```python
from build123d import *

# Parameters (mm, degrees)
F1_DEPTH  = 38.1
F2_W      = 25.4
F2_H      = 38.1
F3_DEPTH  = 25.4
F4_R      = 6.35
F5_DEPTH  = 12.7
F7_DEPTH  = 12.7
F8_W      = 12.7
F8_H      = 12.7
F9_DEPTH  = 12.7
F11_DEPTH = 12.7
F12_R     = 1.5875
F13_DEPTH = 6.35
F15_DEPTH = 6.35


with BuildPart() as f1:
    # F0 (on Front) → F1 (new body)
    with BuildSketch(Plane.XZ):
        Polygon((-17.457331, 44.45), (-42.857331, 44.45), (-42.857331, 0), (26.992669, 0), (26.992669, 6.35), (-17.457331, 6.35), align=None)
    extrude(amount=F1_DEPTH)

    # F2 (on face) → F3 (cut)
    with BuildSketch(Plane.XZ.offset(38.1)):
        with Locations((-30.157331, 25.4)):
            Rectangle(F2_W, F2_H)
    extrude(amount=-F3_DEPTH, mode=Mode.SUBTRACT)

    # F4 (on face) → F5 (cut)
    with BuildSketch(Plane.XZ.offset(12.7)):
        with Locations((-30.157331, 31.75)):
            Circle(F4_R)
    extrude(amount=-F5_DEPTH, mode=Mode.SUBTRACT)

    # F6 (on face) → F7 (cut)
    with BuildSketch(Plane.XZ.offset(12.7)):
        with BuildLine():
            ThreePointArc((-42.857331, 31.75), (-39.137587, 40.730256), (-30.157331, 44.45))
            Line((-30.157331, 44.45), (-42.857331, 44.45))
            Line((-42.857331, 44.45), (-42.857331, 31.75))
        make_face()
        with BuildLine():
            Line((-17.457331, 44.45), (-30.157331, 44.45))
            ThreePointArc((-30.157331, 44.45), (-21.177075, 40.730256), (-17.457331, 31.75))
            Line((-17.457331, 31.75), (-17.457331, 44.45))
        make_face()
    extrude(amount=-F7_DEPTH, mode=Mode.SUBTRACT)

    # F8 (on face) → F9 (join)
    with BuildSketch(Plane.XZ.offset(12.7)):
        with Locations((-11.107331, 12.7)):
            Rectangle(F8_W, F8_H)
    extrude(amount=-F9_DEPTH)

    # F10 (on face) → F11 (cut)
    with BuildSketch(Plane.XZ.offset(12.7)):
        with BuildLine():
            Line((-4.757331, 19.05), (-17.457331, 19.05))
            ThreePointArc((-17.457331, 19.05), (-13.737587, 10.069744), (-4.757331, 6.35))
            Line((-4.757331, 6.35), (-4.757331, 19.05))
        make_face()
    extrude(amount=-F11_DEPTH, mode=Mode.SUBTRACT)

    # F12 (on face) → F13 (cut)
    with BuildSketch(Plane.XY.offset(6.35)):
        with Locations((-33.332331, -28.575)):
            Circle(F12_R)
        with Locations((17.467669, -28.575)):
            Circle(F12_R)
        with Locations((17.467669, -9.525)):
            Circle(F12_R)
    extrude(amount=-F13_DEPTH, mode=Mode.SUBTRACT)

    # F14 (on face) → F15 (cut)
    with BuildSketch(Plane.XY.offset(6.35)):
        with BuildLine():
            ThreePointArc((-30.157331, -38.1), (-39.137587, -34.380256), (-42.857331, -25.4))
            Line((-42.857331, -25.4), (-42.857331, -38.1))
            Line((-42.857331, -38.1), (-30.157331, -38.1))
        make_face()
        with BuildLine():
            ThreePointArc((26.992669, -25.4), (23.272925, -34.380256), (14.292669, -38.1))
            Line((14.292669, -38.1), (26.992669, -38.1))
            Line((26.992669, -38.1), (26.992669, -25.4))
        make_face()
    extrude(amount=-F15_DEPTH, mode=Mode.SUBTRACT)


solid = f1.part
```
Read the model definition and answer for the solid it produces. Units are mm, in the model's axes. A direction names the side the tool comes from. Coordinates: 2 decimals unless noted, no trailing zeros. Write each loop counter-clockwise with the first axis right and the second up, starting at its lowest first coordinate (ties: lowest second). Pieces come first, ordered by that corner, then holes. Notation, with made-up numbers: (31, 31) -> (51, 31) arc R19 cw to (51, 57) -> close; hole circle Ø2 at (-5, -15.75). An arc over 180 degrees is marked (long way). Answer as a JSON object with one key per item and string values.
Q1. The part is cut by section B-B on y = -24. Give the vertices of the cut face in (x, z).
The answers:
{"outline": "(-42.86, 0) -> (26.99, 0) -> (26.99, 6.35) -> (-42.86, 6.35) -> close"}
Q2. Determine the mould class of faces 6 (the flat face through (-24, 0, 18)), 7 (the cylindrical face through (-24.1, -6.44, 33.66)), 8 (the cylindrical face through (-13.836, -6.439, 10.169)), 9 (the cylindrical face through (-39.038, -34.478, 3.219)) for opening direction X: pulls with the +X half, pulls with the -X half, needs draft (parallel to the pull), parting line crosses it, or undercut.
The answers:
{"face 6": "needs draft", "face 7": "undercut", "face 8": "pulls with the +X half", "face 9": "pulls with the -X half"}
Q3. A tool of negligible diameter and unlimited length cuts with its end or side. For faces 1 (the flat face through (-42.857, -10, 13)), 2 (the flat face through (-7, -23, 6.35)), 3 (the flat face through (26.993, -13, 3)), 4 (the flat face through (-28, -12.7, 21)), 5 (the flat face through (-17.457, -6, 25)), from which of +Z, -Z, +X, -X, +Y, -Y can it reach the whole face along a straight path? Write none if from no direction.
The answers:
{"face 1": "+Z, -Z, -X, +Y, -Y", "face 2": "+Z, +X, -Y", "face 3": "+Z, -Z, +X, +Y, -Y", "face 4": "+Z, +X, -X, -Y", "face 5": "+Z, +X, +Y, -Y"}
Q4. Consider line 1 (X direction, y = -6.5, z = 32); line 2 (Y direction, x = -38, z = 38); line 3 (Z direction, x = -27.5, y = -13). Determine where each line is inside the solid, lowest interval first. Write a range as [from, to].
The answers:
{"line 1": "x = [-42.85, -36.5], [-23.81, -17.46]", "line 2": "y = [-12.7, 0]", "line 3": "z = [0, 6.35]"}
Q5. Flat-ended cylindrical pins translate along their axes: pin 1 Ø2 at (x, z) = (4, 9) entering from -Y; pin 2 Ø6 at (x, y) = (-6, -30.5) entering from +Z; pin 3 Ø3 at (x, y) = (-1.5, -23.5) entering from +Z; pin 4 Ø4 at (y, z) = (-4, 25) entering from +X. Find the tip coordinate at first contact, or state that the pin passes through.
The answers:
{"pin 1": "passes through", "pin 2": "stops at z = 6.35", "pin 3": "stops at z = 6.35", "pin 4": "stops at x = -17.46"}
Q6. The part is cut by section D-D on x = -7. Give the vertices of the cut face in (y, z), then the cut area to 3 significant figures.
The answers:
{"outline": "(-38.1, 0) -> (0, 0) -> (0, 6.55) -> (-12.7, 6.55) -> (-12.7, 6.35) -> (-38.1, 6.35) -> close", "area": "244 mm2"}
Q7. The part is cut by section C-C on z = 34. Give the vertices of the cut face in (x, y), then the cut area to 3 significant figures.
The answers:
{"outline": "(-42.66, -12.7) -> (-36.1, -12.7) -> (-36.1, 0) -> (-42.66, 0) -> close; (-24.22, -12.7) -> (-17.66, -12.7) -> (-17.66, 0) -> (-24.22, 0) -> close", "area": "167 mm2"}
Q8. The part is cut by section A-A on z = 3. Give the vertices of the cut face in (x, y) (1 decimal).
The answers:
{"outline": "(-42.9, -25.4) arc R12.7 ccw to (-30.2, -38.1) -> (14.3, -38.1) arc R12.7 ccw to (27, -25.4) -> (27, 0) -> (-42.9, 0) -> close; hole circle Ø3.2 at (-33.3, -28.6); hole circle Ø3.2 at (17.5, -28.6); hole circle Ø3.2 at (17.5, -9.5)"}
